Read the model definition and answer for the solid it produces. Units are mm, in the model's axes. A direction names the side the tool comes from. Give positions to 0.01 mm unless a question says otherwise; leave off trailing zeros. Loops run counter-clockwise (first coordinate to the right, second up) from the corner with the lowest first, then second, coordinate; pieces in that order, holes last. Notation, with made-up numbers: (34.5, -28) -> (67.5, -28) arc R10 ccw to (67.5, -17) -> close; hole circle Ø5 at (1, 40.25). An arc over 180 degrees is marked (long way). Answer as CSV lines item,"result". Start each with the question number.
```python
from build123d import *

# Parameters (mm, degrees)
SKETCH2_W               = 150
SKETCH2_H               = 50
BOSS_EXTRUDE1_DEPTH     = 50
SKETCH5_W               = 30
SKETCH5_H               = 30
CUT_EXTRUDE1_DEPTH      = 1
CUT_EXTRUDE1_DEPTH_BACK = 151
SKETCH7_R               = 55.901699437
SKETCH7_R_2             = 15
SKETCH7_R_3             = 5
BOSS_EXTRUDE2_DEPTH     = 20
BOSS_EXTRUDE3_START     = -3
BOSS_EXTRUDE3_DEPTH     = 6.25
SKETCH11_R              = 5
CUT_EXTRUDE2_DEPTH      = 31.901699437
CUT_EXTRUDE2_DEPTH_BACK = 81.901699437


with BuildPart() as part:
    # Sketch2 → Boss-Extrude1 (new body)
    with BuildSketch(Plane(origin=(0, 0, 0), x_dir=(1, 0, 0), z_dir=(0, 1, 0))):
        Rectangle(SKETCH2_W, SKETCH2_H)
    extrude(amount=BOSS_EXTRUDE1_DEPTH)

    # Sketch5 → Cut-Extrude1 (cut, two sides)
    with BuildSketch(Plane(origin=(75, 0, 0), x_dir=(0, 0, -1), z_dir=(1, 0, 0))) as cut_extrude1_sk:
        with Locations((0, 25)):
            Rectangle(SKETCH5_W, SKETCH5_H)
    extrude(amount=CUT_EXTRUDE1_DEPTH, mode=Mode.SUBTRACT)
    extrude(cut_extrude1_sk.sketch, amount=-CUT_EXTRUDE1_DEPTH_BACK, mode=Mode.SUBTRACT)

    # Sketch7 → Boss-Extrude2 (add)
    with BuildSketch(Plane(origin=(75, 0, 0), x_dir=(0, 0, -1), z_dir=(1, 0, 0))):
        with Locations((0, 100)):
            Circle(SKETCH7_R)
        with Locations((0, 100)):
            Circle(SKETCH7_R_2, mode=Mode.SUBTRACT)
        with Locations((0, 132.030384042)):
            Circle(SKETCH7_R_3, mode=Mode.SUBTRACT)
        with Locations((32.030384042, 100)):
            Circle(SKETCH7_R_3, mode=Mode.SUBTRACT)
        with Locations((0, 67.969615958)):
            Circle(SKETCH7_R_3, mode=Mode.SUBTRACT)
        with Locations((-32.030384042, 100)):
            Circle(SKETCH7_R_3, mode=Mode.SUBTRACT)
    extrude(amount=-BOSS_EXTRUDE2_DEPTH)

    # Sketch8 → Boss-Extrude3 (add)
    with BuildSketch(Plane(origin=(0, 0, -25), x_dir=(-1, 0, 0), z_dir=(0, 0, -1)).offset(BOSS_EXTRUDE3_START)):
        Polygon((75, 50), (-55, 151.408233922), (-55, 50), align=None)
    boss_extrude3 = extrude(amount=-BOSS_EXTRUDE3_DEPTH)

    # Sketch11 → Cut-Extrude2 (cut, two sides)
    with BuildSketch(Plane.XY.offset(25)) as cut_extrude2_sk:
        with Locations((0, 25)):
            Circle(SKETCH11_R)
    extrude(amount=CUT_EXTRUDE2_DEPTH, mode=Mode.SUBTRACT)
    extrude(cut_extrude2_sk.sketch, amount=-CUT_EXTRUDE2_DEPTH_BACK, mode=Mode.SUBTRACT)

    # Mirror1: Boss-Extrude3 across plane
    add(boss_extrude3.mirror(Plane.XY))


solid = part.part
```
(1) Each of these flat-tipped pins is pushed along its axis until it touches: P1, Ø4, axis at x = -55.5, y = 17.5, coming from the -Z side; P2, Ø4, axis at y = 58, z = 3, coming from the -X side; P3, Ø12, axis at x = 48, y = 89.5, coming from the +Z side. Where does it stop, or does it pass through?
(2) Find section B-B on z = 0. Write down the section's boundary in (x, y), then the cut area to 3 significant figures.
(3) Find the intervals of material crossed by line 1 along Y through (x, z) = (66, 0); line 2 along Z through (x, y) = (25, 20); line 3 along Z through (x, y) = (4.5, 54), in increasing order. Write a range as from..to.
(4) Find section D-D on y = 129. Write down the section's boundary in (x, z).
(5) The mould has two halves that part along Y. Classify faces 4 (the face through (-1, 19, -25)), 5 (the face through (-10.9, 100, 18.9)), 6 (the face through (-1.08, 20.12, 20.07)): pulls with the +Y half, pulls with the -Y half, needs draft (parallel to the pull), parting line crosses it, or undercut.
(6) Find section C-C on x = 0. Write down the section's boundary in (y, z).
(7) Find section A-A on y = 25. Write down the section's boundary in (x, z).
(8) A tool of negligible diameter and unlimited length cuts with its end or side. For faces 1 (the face through (55, 115.5, 0.3)), 2 (the face through (20, 79, -22)), 3 (the face through (1, 31, -15)), from which of +Z, -Z, +X, -X, +Y, -Y can it reach the whole face along a straight path? Write none if from no direction.
Answer block:
1,P1,"stops at z = -25"
1,P2,"stops at x = 55"
1,P3,"stops at z = 22"
2,outline,"(-75, 0) -> (75, 0) -> (75, 10) -> (-75, 10) -> close; (-75, 40) -> (75, 40) -> (75, 62.97) -> (55, 62.97) -> (55, 50) -> (-75, 50) -> close; (55, 72.97) -> (75, 72.97) -> (75, 85) -> (55, 85) -> close; (55, 115) -> (75, 115) -> (75, 127.03) -> (55, 127.03) -> close; (55, 137.03) -> (75, 137.03) -> (75, 155.9) -> (55, 155.9) -> close"
2,area,"4,120 mm2"
3,line 1,"y = 0..10, 40..62.97, 72.97..85, 115..127.03, 137.03..155.9"
3,line 2,"z = -25..-15, 15..25"
3,line 3,"z = -22..-15.75, 15.75..22"
4,outline,"(26.27, -22) -> (55, -22) -> (55, -47.79) -> (75, -47.79) -> (75, -3.98) -> (55, -3.98) -> (55, -15.75) -> (26.27, -15.75) -> close; (26.27, 15.75) -> (55, 15.75) -> (55, 3.98) -> (75, 3.98) -> (75, 47.79) -> (55, 47.79) -> (55, 22) -> (26.27, 22) -> close"
5,face 4,"needs draft"
5,face 5,"pulls with the +Y half"
5,face 6,"undercut"
6,outline,"(0, -25) -> (20, -25) -> (20, -15) -> (10, -15) -> (10, 15) -> (20, 15) -> (20, 25) -> (0, 25) -> close; (30, -25) -> (50, -25) -> (50, -22) -> (108.5, -22) -> (108.5, -15.75) -> (50, -15.75) -> (50, 15.75) -> (108.5, 15.75) -> (108.5, 22) -> (50, 22) -> (50, 25) -> (30, 25) -> (30, 15) -> (40, 15) -> (40, -15) -> (30, -15) -> close"
7,outline,"(-75, -25) -> (-5, -25) -> (-5, -15) -> (-75, -15) -> close; (-75, 15) -> (-5, 15) -> (-5, 25) -> (-75, 25) -> close; (5, -25) -> (75, -25) -> (75, -15) -> (5, -15) -> close; (5, 15) -> (75, 15) -> (75, 25) -> (5, 25) -> close"
8,face 1,"-X, +Y"
8,face 2,"-Z, -X, +Y"
8,face 3,"+X, -X"
